For this review, take the finished solid that the model builds, in its own axes (mm). A direction names the side the tool comes from. Coordinates: 2 decimals unless noted, no trailing zeros. Loops run counter-clockwise (first coordinate to the right, second up) from the corner with the lowest first, then second, coordinate; pieces in that order, holes last. Notation, with made-up numbers: (85.5, 64) -> (131.5, 64) arc R20 cw to (131.5, 68) -> close; hole circle Ø5 at (-22, 55). An arc over 180 degrees is marked (long way). Answer in a Markdown table with one row per item.
from build123d import *

# Parameters (mm, degrees)
F0_R     = 15
F1_DEPTH = 20
F2_R     = 20
F3_DEPTH = 200
F4_W     = 165
F4_H     = 8
F5_DEPTH = 25
F7_D     = 10
F7_DEPTH = 20.001
F8_R     = 15
F9_DEPTH = 10


with BuildPart() as f1:
    # F0 (on Right) → F1 (new body)
    with BuildSketch(Plane.YZ):
        Circle(F0_R)
    extrude(amount=F1_DEPTH)

    # F2 (on face) → F3 (join)
    with BuildSketch(Plane.YZ.offset(20)):
        Circle(F2_R)
    extrude(amount=F3_DEPTH)

    # F4 (on Top) → F5 (cut, symmetric)
    with BuildSketch(Plane.XY):
        with Locations((127.5, -4)):
            Rectangle(F4_W, F4_H)
    extrude(amount=F5_DEPTH, both=True, mode=Mode.SUBTRACT)

    # F7 (through all, one way)
    with BuildSketch(Plane(origin=(0, 0, 0), x_dir=(1, 0, 0), z_dir=(0, 1, 0))):
        with Locations((60, 0), (85, 0), (110, 0), (135, 0), (160, 0), (185, 0)):
            Circle(F7_D / 2)
    extrude(amount=-F7_DEPTH, mode=Mode.SUBTRACT)

    # F8 (on face) → F9 (join)
    with BuildSketch(Plane.YZ.offset(220)):
        Circle(F8_R)
    extrude(amount=F9_DEPTH)


solid = f1.part
Item 1: For L1, parallel to X at y = -1, z = -9; L2, parallel to X at y = 13.5, z = 10; L3, parallel to Y at x = 114.5, z = -3, list the stretches that pass through material, from the lowest coordinate up.
Worked answers:
| item | result |
|---|---|
| L1 | 0 to 45, 210 to 230 |
| L2 | 20 to 220 |
| L3 | -19.77 to -8, 0 to 19.77 |
Item 2: Take a section at C-C, the plane x = 78. State the section outline as (y, z) points, and give its area (3 significant figures).
Worked answers:
| item | result |
|---|---|
| outline | (-8, -18.33) -> (-8, 18.33) arc R20 ccw to start; (0, -20) arc R20 ccw to (0, 20) -> close |
| area | 945 mm² |
Item 3: Take a section at D-D, the plane x = 135. State the section outline as (y, z) points, and give its area (3 significant figures).
Worked answers:
| item | result |
|---|---|
| outline | (-19.36, -5) arc R20 ccw to (-8, -18.33) -> (-8, -5) -> close; (-19.36, 5) -> (-8, 5) -> (-8, 18.33) arc R20 ccw to start; (0, -20) arc R20 ccw to (0, 20) -> close |
| area | 827 mm² |
Item 4: Take a section at A-A, the plane y = -6. State the section outline as (x, z) points.
Worked answers:
| item | result |
|---|---|
| outline | (0, -13.75) -> (20, -13.75) -> (20, -19.08) -> (45, -19.08) -> (45, 19.08) -> (20, 19.08) -> (20, 13.75) -> (0, 13.75) -> close; (210, -19.08) -> (220, -19.08) -> (220, -13.75) -> (230, -13.75) -> (230, 13.75) -> (220, 13.75) -> (220, 19.08) -> (210, 19.08) -> close |
Item 5: The part is to be moulded in two halves that separate along Y. For faces 1 (the flat face through (45, -4, 0)), 2 (the cylindrical face through (114.619, -13.916, 1.915)), 3 (the flat face through (126, -8, 0)), 4 (the cylindrical face through (118.6, 19.076, 6.007)), say which applies: +Y half, -Y half, draft (parallel to the pull), parting line (faces both ways), or undercut.
Worked answers:
| item | result |
|---|---|
| face 1 | undercut |
| face 2 | draft |
| face 3 | undercut |
| face 4 | parting line |
Item 6: For faces 5 (the flat face through (220, 3, 15)), 6 (the flat face through (20, 3, 15)), 7 (the cylindrical face through (139.77, -13.92, -1.5)), 8 (the flat face through (210, -4, 0)), list the 3-axis set-ups (+Z, -Z, +X, -X, +Y, -Y) from which the entire face can be reached by the end or side of a thin tool; tool diameter is ignored.
Worked answers:
| item | result |
|---|---|
| face 5 | +X |
| face 6 | -X |
| face 7 | -Y |
| face 8 | +Z, -Z |
Item 7: Insertion check: pin 1 (12 mm diameter, centred on y = -7, z = -10.5, fed in from -X); pin 2 (4 mm diameter, centred on x = 142, y = 12.5, fed in from -Z); pin 3 (4 mm diameter, centred on y = 15.5, z = -8, fed in from +X); pin 4 (1.5 mm diameter, centred on x = 202.5, z = 5.5, fed in from +Y). Each pin has a flat end and moves straight along its axis. Give the tip position at first contact, or say it passes through.
Worked answers:
| item | result |
|---|---|
| pin 1 | x = 0 |
| pin 2 | z = -17.02 |
| pin 3 | x = 220 |
| pin 4 | y = 19.43 |
Item 8: Take a section at B-B, the plane z = 0. Count the separate pieces of the cut face and the enclosed holes in it, and give its area (3 significant figures).
Worked answers:
| item | result |
|---|---|
| separate pieces | 6 |
| enclosed holes | 0 |
| area | 6,860 mm² |
